Work out the finished part from the listing and answer in its coordinate system (mm). A direction names the side the tool comes from. Give positions to 0.01 mm unless a question says otherwise; leave off trailing zeros. Order: outer loops, then holes, each group sorted by start corner. A loop starts at its lowest first (then second) coordinate and runs counter-clockwise, first axis right, second up.
```python
from build123d import *

# Parameters (mm, degrees)
BOSS_EXTRUDE1_DEPTH     = 5
BOSS_EXTRUDE2_DEPTH     = 3
BOSS_EXTRUDE3_DEPTH     = 3
SKETCH10_W              = 9.5
SKETCH10_H              = 5
BOSS_EXTRUDE4_DEPTH     = 15.78
SKETCH11_W              = 9.5
SKETCH11_H              = 2
BOSS_EXTRUDE5_DEPTH     = 40
BOSS_EXTRUDE6_DEPTH     = 6.09393
SKETCH14_R              = 1.8
CUT_EXTRUDE1_DEPTH      = 6.3
SKETCH15_W              = 51.153217575
SKETCH15_H              = 86.05062267
CUT_EXTRUDE3_DEPTH      = 6
CUT_EXTRUDE3_DEPTH_BACK = 19.78
SKETCH16_W              = 9.603970124
SKETCH16_H              = 11.884913028
CUT_EXTRUDE4_DEPTH      = 17.733728816


with BuildPart() as part:
    # Sketch3 → Revolve1 (revolve)
    with BuildSketch(Plane.XY):
        Polygon((-62.694264441, 10.250679103), (-62.694264441, 11.733728816), (-64.884531744, 11.733728816), (-64.884531744, 5.639799249), (-60.884531744, 5.639799249), (-60.884531744, 6.650679103), (-62.694264441, 6.650679103), align=None)
    revolve(axis=Axis((-49.744264441, 0, 0), (0, 1, 0)))

    # Sketch7 → Boss-Extrude1 (add)
    with BuildSketch(Plane(origin=(0, 11.733728816, 0), x_dir=(1, 0, 0), z_dir=(0, 1, 0))):
        with BuildLine():
            Line((-50.244264441, 15.132008921), (-50.244264441, 12.94034389))
            ThreePointArc((-50.244264441, 12.94034389), (-49.744264441, 12.95), (-49.244264441, 12.94034389))
            Line((-49.244264441, 12.94034389), (-49.244264441, 15.132008921))
            ThreePointArc((-49.244264441, 15.132008921), (-49.744264441, 15.140267302), (-50.244264441, 15.132008921))
        make_face()
    extrude(amount=BOSS_EXTRUDE1_DEPTH)

    # Sketch8 → Boss-Extrude2 (add)
    with BuildSketch(Plane(origin=(0, 16.733728816, 0), x_dir=(1, 0, 0), z_dir=(0, 1, 0))):
        with BuildLine():
            Line((-50.244264441, 15.132008921), (-50.244264441, 12.94034389))
            Line((-50.244264441, 12.94034389), (-50.244264441, -4.55965611))
            Line((-50.244264441, -4.55965611), (-49.244264441, -4.55965611))
            Line((-49.244264441, -4.55965611), (-49.244264441, 12.94034389))
            Line((-49.244264441, 12.94034389), (-49.244264441, 15.132008921))
            ThreePointArc((-49.244264441, 15.132008921), (-49.744264441, 15.140267302), (-50.244264441, 15.132008921))
        make_face()
    extrude(amount=-BOSS_EXTRUDE2_DEPTH)

    # Sketch9 → Boss-Extrude3 (add)
    with BuildSketch(Plane(origin=(0, 11.733728816, 0), x_dir=(1, 0, 0), z_dir=(0, 1, 0))):
        with BuildLine():
            Line((-54.494264441, 14.375854548), (-54.494264441, 39.375854548))
            Line((-54.494264441, 39.375854548), (-44.994264441, 39.375854548))
            Line((-44.994264441, 39.375854548), (-44.994264441, 14.375854548))
            ThreePointArc((-44.994264441, 14.375854548), (-47.092177082, 14.906177465), (-49.244264441, 15.132008921))
            ThreePointArc((-49.244264441, 15.132008921), (-49.744264441, 15.140267302), (-50.244264441, 15.132008921))
            ThreePointArc((-50.244264441, 15.132008921), (-52.3963518, 14.906177465), (-54.494264441, 14.375854548))
        make_face()
    extrude(amount=-BOSS_EXTRUDE3_DEPTH)

    # Sketch10 → Boss-Extrude4 (add)
    with BuildSketch(Plane.XZ.offset(-8.733728816)):
        with Locations((-49.744264441, -36.875854548)):
            Rectangle(SKETCH10_W, SKETCH10_H)
    extrude(amount=BOSS_EXTRUDE4_DEPTH)

    # Sketch11 → Boss-Extrude5 (add)
    with BuildSketch(Plane(origin=(0, 0, -39.375854548), x_dir=(-1, 0, 0), z_dir=(0, 0, -1))):
        with Locations((49.744264441, -6.046271184)):
            Rectangle(SKETCH11_W, SKETCH11_H)
    extrude(amount=BOSS_EXTRUDE5_DEPTH)

    # Sketch13 → Boss-Extrude6 (add)
    with BuildSketch(Plane(origin=(0, 11.733728816, 0), x_dir=(1, 0, 0), z_dir=(0, 1, 0))):
        with BuildLine():
            Line((-28.603997139, 3.15), (-34.935307895, 3.15))
            ThreePointArc((-34.935307895, 3.15), (-34.603997139, 0), (-34.935307895, -3.15))
            Line((-34.935307895, -3.15), (-28.603997139, -3.15))
            Line((-28.603997139, -3.15), (-28.603997139, 3.15))
        make_face()
        with BuildLine():
            Line((-70.884531744, 3.15), (-70.884531744, -3.15))
            Line((-70.884531744, -3.15), (-64.553220987, -3.15))
            ThreePointArc((-64.553220987, -3.15), (-64.884531744, 0), (-64.553220987, 3.15))
            Line((-64.553220987, 3.15), (-70.884531744, 3.15))
        make_face()
    extrude(amount=-BOSS_EXTRUDE6_DEPTH)

    # Sketch14 → Cut-Extrude1 (cut)
    with BuildSketch(Plane.XY.offset(3.15)):
        with Locations((-31.769652517, 8.686764033)):
            Circle(SKETCH14_R)
        with Locations((-67.718876365, 8.686764033)):
            Circle(SKETCH14_R)
    extrude(amount=-CUT_EXTRUDE1_DEPTH, mode=Mode.SUBTRACT)

    # Sketch15 → Cut-Extrude3 (cut, two sides)
    with BuildSketch(Plane(origin=(0, 11.733728816, 0), x_dir=(1, 0, 0), z_dir=(0, 1, 0))) as cut_extrude3_sk:
        with Locations((-49.018725857, 43.025311335)):
            Rectangle(SKETCH15_W, SKETCH15_H)
    extrude(amount=CUT_EXTRUDE3_DEPTH, mode=Mode.SUBTRACT)
    extrude(cut_extrude3_sk.sketch, amount=-CUT_EXTRUDE3_DEPTH_BACK, mode=Mode.SUBTRACT)

    # Sketch16 → Cut-Extrude4 (cut, through all)
    with BuildSketch(Plane(origin=(0, 0, 0), x_dir=(1, 0, 0), z_dir=(0, 1, 0))):
        with Locations((-50.086315959, -0.525030424)):
            Rectangle(SKETCH16_W, SKETCH16_H)
    extrude(amount=CUT_EXTRUDE4_DEPTH, mode=Mode.SUBTRACT)


solid = part.part
```
1. Given P1, Ø2, axis at y = 9.5, z = 12.5, coming from the +X side; P2, Ø3, axis at y = 9.5, z = 8.5, coming from the -X side; P3, Ø3, axis at x = -31, y = 9.5, coming from the +Z side, each flat-ended and moving along its own axis, determine where each tip first touches the part or whether it passes through.
Findings below:
P1: stops at x = -39.9
P2: stops at x = -63.17
P3: stops at z = 3.15
2. The part is cut by section A-A (z = 2.5). Write down the section's boundary in (x, y), then the cut area to 3 significant figures.
Findings below:
outline: (-70.88, 5.64) - (-60.6, 5.64) - (-60.6, 6.65) - (-62.45, 6.65) - (-62.45, 11.73) - (-70.88, 11.73) - close; (-38.89, 5.64) - (-28.6, 5.64) - (-28.6, 11.73) - (-37.04, 11.73) - (-37.04, 6.65) - (-38.89, 6.65) - close; hole circle Ø3.6 at (-67.72, 8.69); hole circle Ø3.6 at (-31.77, 8.69)
area: 86.2 mm2
3. The part is cut by section D-D (z = 11.75). Write down the section's boundary in (x, y), then the cut area to 3 significant figures.
Findings below:
outline: (-59.29, 5.64) - (-40.2, 5.64) - (-40.2, 11.73) - (-44.3, 11.73) - (-44.3, 6.65) - (-55.19, 6.65) - (-55.19, 11.73) - (-59.29, 11.73) - close
area: 61.0 mm2
4. Straight lines are drawn through the part: probe 1 along Y at (x, z) = (-57, 10.5); probe 2 along X at (y, z) = (6.75, 8.5); probe 3 along X at (y, z) = (10, 9.25). For each, find the intervals that lie inside material, in ascending order.
Findings below:
probe 1: y = 5.64 to 6.65
probe 2: x = -62.27 to -59.51, -39.97 to -37.22
probe 3: x = -61.73 to -58.81, -40.68 to -37.76
5. Which of the six approach directions +Z, -Z, +X, -X, +Y, -Y give full straight-line access (tool end or side, diameter ignored) to faces 1 (the face through (-53, 11.734, 13)), 2 (the face through (-66, 7, 3.15)), 3 (the face through (-50.029, 9.228, 12.947))?
Findings below:
face 1: +Z, -Z, +X, -X, +Y
face 2: +Z, -X, +Y, -Y
face 3: -Z, +Y
6. The part is cut by section C-C (x = -40). Write down the section's boundary in (y, z), then the cut area to 3 significant figures.
Findings below:
outline: (5.64, 5.4) - (6.65, 5.4) - (6.65, 8.53) - (11.73, 8.53) - (11.73, 11.59) - (5.64, 11.59) - close
area: 21.8 mm2
7. The part is cut by section B-B (y = 11). Write down the section's boundary in (x, z).
Findings below:
outline: (-70.88, 0) - (-62.69, 0) arc R12.95 cw to (-36.79, 0) - (-28.6, 0) - (-28.6, 3.15) - (-34.94, 3.15) arc R15.14 ccw to (-64.55, 3.15) - (-70.88, 3.15) - close
8. The mould has two halves that part along X. Classify faces 4 (the face through (-49.8, 6.651, 11.3)), 5 (the face through (-28.604, 9, 2)), 6 (the face through (-30, 7, 3.15)), 7 (the face through (-70.885, 9, 2)): pulls with the +X half, pulls with the -X half, needs draft (parallel to the pull), parting line crosses it, or undercut.
Findings below:
face 4: undercut
face 5: pulls with the +X half
face 6: needs draft
face 7: pulls with the -X half
